```python
from build123d import *

# Parameters (mm, degrees)
BOSS_EXTRUDE1_DEPTH     = 47.498
CUT_EXTRUDE3_DEPTH      = 115.467517244
CUT_EXTRUDE3_DEPTH_BACK = 115.467517244
SKETCH2_R               = 2.413
SKETCH2_4_R             = 2.413
CUT_EXTRUDE4_DEPTH      = 115.467517244
SKETCH6_R               = 12.7
BOSS_EXTRUDE5_DEPTH     = 25.4
SKETCH6_6_R             = 12.7
BOSS_EXTRUDE6_DEPTH     = 25.4
SKETCH8_R               = 2.413
CUT_EXTRUDE5_DEPTH      = 25.4
SKETCH9_R               = 2.413
CUT_EXTRUDE6_DEPTH      = 25.4


with BuildPart() as part:
    # Sketch1 → Boss-Extrude1 (new body)
    with BuildSketch(Plane(origin=(0, 0, 0), x_dir=(1, 0, 0), z_dir=(0, 1, 0))):
        with BuildLine():
            Line((0, 0), (0, 63.5))
            Line((0, 63.5), (12.7, 63.5))
            ThreePointArc((12.7, 63.5), (41.275, 34.925), (69.85, 63.5))
            Line((69.85, 63.5), (82.55, 63.5))
            Line((82.55, 63.5), (82.55, 0))
            Line((82.55, 0), (0, 0))
        make_face()
    extrude(amount=BOSS_EXTRUDE1_DEPTH)

    # Sketch2 → Cut-Extrude3 (cut, two sides: drawn at the far end of the back side and taken through both)
    with BuildSketch(Plane(origin=(0, 47.498, 0), x_dir=(1, 0, 0), z_dir=(0, 1, 0)).offset(-CUT_EXTRUDE3_DEPTH_BACK)):
        with Locations(Location((15.875, 12.7, 0), (0, 0, 90))):
            Circle(SKETCH2_R)
    extrude(amount=CUT_EXTRUDE3_DEPTH + CUT_EXTRUDE3_DEPTH_BACK, mode=Mode.SUBTRACT)

    # Sketch2_4 → Cut-Extrude4 (cut, through all)
    with BuildSketch(Plane(origin=(0, 47.498, 0), x_dir=(1, 0, 0), z_dir=(0, 1, 0))):
        with Locations(Location((15.875, 12.7, 0), (0, 0, 90))):
            Circle(SKETCH2_4_R)
        with Locations(Location((41.275, 12.7, 0), (0, 0, 270))):
            Circle(SKETCH2_4_R)
        with Locations(Location((66.675, 12.7, 0), (0, 0, 270))):
            Circle(SKETCH2_4_R)
    extrude(amount=-CUT_EXTRUDE4_DEPTH, mode=Mode.SUBTRACT)

    # Sketch6 → Boss-Extrude5 (add)
    with BuildSketch(Plane(origin=(0, 0, -63.5), x_dir=(-1, 0, 0), z_dir=(0, 0, -1))):
        with Locations((-82.55, 23.749)):
            Circle(SKETCH6_R)
    extrude(amount=-BOSS_EXTRUDE5_DEPTH)

    # Sketch6_6 → Boss-Extrude6 (add)
    with BuildSketch(Plane(origin=(0, 0, -63.5), x_dir=(-1, 0, 0), z_dir=(0, 0, -1))):
        with Locations((0, 24.290625464)):
            Circle(SKETCH6_6_R)
        with Locations((-82.55, 23.749)):
            Circle(SKETCH6_6_R)
    extrude(amount=-BOSS_EXTRUDE6_DEPTH)

    # Sketch8 → Cut-Extrude5 (cut)
    with BuildSketch(Plane(origin=(0, 0, -63.5), x_dir=(-1, 0, 0), z_dir=(0, 0, -1))):
        with Locations((-88.9, 23.749)):
            Circle(SKETCH8_R)
    extrude(amount=-CUT_EXTRUDE5_DEPTH, mode=Mode.SUBTRACT)

    # Sketch9 → Cut-Extrude6 (cut)
    with BuildSketch(Plane(origin=(0, 0, -63.5), x_dir=(-1, 0, 0), z_dir=(0, 0, -1))):
        with Locations((6.296749676, 24.139451287)):
            Circle(SKETCH9_R)
    extrude(amount=-CUT_EXTRUDE6_DEPTH, mode=Mode.SUBTRACT)


solid = part.part
```
Source: CAD feature listing. Evaluate the final solid. Frame: model axes, mm. A direction names the side the tool comes from. Round coordinates to 2 decimals unless told otherwise and drop trailing zeros. Loops run counter-clockwise (first coordinate to the right, second up) from the corner with the lowest first, then second, coordinate; pieces in that order, holes last. Notation, with made-up numbers: M 13.5,-26 L 41.5,-26 A31 ccw 41.5,12 Z; hole C 1.5,77.25 d4. An arc over 180 degrees is marked long. Use a Markdown table: item, result. Add a question column.
1. Line query: line 1 (X direction, y = 30, z = -12.7); line 2 (X direction, y = 2.5, z = -5.5); line 3 (Z direction, x = 17, y = 32). Output: solid intervals per line, ascending.
2. Contact query for flat-ended pins moving along their axis: P1, Ø10, axis at x = 13.5, y = 24.5, coming from the -Z side; P2, Ø14, axis at y = 15, z = -44, coming from the -X side; P3, Ø1.5, axis at y = 37, z = -22, coming from the -X side; P4, Ø10, axis at y = 24, z = -9, coming from the +X side. Output: stop coordinate, or through.
3. Reachability of faces 4 (the flat face through (82.55, 23, -25)), 5 (the flat face through (0, 23, -24)), 6 (the flat face through (-3, 24, -38.1)), 7 (the flat face through (86, 24, -38.1)) from +Z, -Z, +X, -X, +Y, -Y: full face, straight path, thin tool, end or side. Return the list, or none.
4. Mould query, pull axis X, two halves, no side actions, for faces 1 (the flat face through (42, 0, -25)), 2 (the cylindrical face through (95.247, 24.028, -50.978)), 3 (the cylindrical face through (-4.52, 25.77, -50.98)). Classes: pulls with the +X half, pulls with the -X half, needs draft (parallel to the pull), parting line crosses it, or undercut.
5. Section query D-D on y = 45. Return the cut outline in (x, z) (3 decimals), then the cut area to 3 significant figures.
6. Section query A-A on z = -12.7. Return the cut outline in (x, y).
7. Section query C-C on x = 88.9. Return the cut outline in (y, z), then the cut area to 3 significant figures.
8. Section query B-B on z = -45.5. Return the cut outline in (x, y).
Reported:
| question | item | result |
|---|---|---|
| 1 | line 1 | x = 0 to 13.46, 18.29 to 38.86, 43.69 to 64.26, 69.09 to 82.55 |
| 1 | line 2 | x = 0 to 82.55 |
| 1 | line 3 | z = -48.43 to -14.83, -10.57 to 0 |
| 2 | P1 | stops at z = -63.5 |
| 2 | P2 | stops at x = -12.49 |
| 2 | P3 | stops at x = 0 |
| 2 | P4 | stops at x = 82.55 |
| 3 | face 4 | +Z, +X |
| 3 | face 5 | +Z, -X |
| 3 | face 6 | +Z, -X, +Y, -Y |
| 3 | face 7 | +Z, +X, +Y, -Y |
| 4 | face 1 | needs draft |
| 4 | face 2 | pulls with the +X half |
| 4 | face 3 | undercut |
| 5 | outline | M 0,-63.5 L 12.7,-63.5 A28.575 cw 69.85,-63.5 L 82.55,-63.5 L 82.55,0 L 0,0 Z; hole C 15.875,-12.7 d4.826; hole C 41.275,-12.7 d4.826; hole C 66.675,-12.7 d4.826 |
| 5 | area | 3,900 mm² |
| 6 | outline | M 0,0 L 13.46,0 L 13.46,47.5 L 0,47.5 Z; M 18.29,0 L 38.86,0 L 38.86,47.5 L 18.29,47.5 Z; M 43.69,0 L 64.26,0 L 64.26,47.5 L 43.69,47.5 Z; M 69.09,0 L 82.55,0 L 82.55,47.5 L 69.09,47.5 Z |
| 7 | outline | M 12.75,-63.5 L 21.34,-63.5 L 21.34,-38.1 L 12.75,-38.1 Z; M 26.16,-63.5 L 34.75,-63.5 L 34.75,-38.1 L 26.16,-38.1 Z |
| 7 | area | 436 mm² |
| 8 | outline | M 0,0 L 19.08,0 L 19.08,47.5 L 0,47.5 L 0,36.99 A12.7 ccw 0,11.59 Z; M 63.47,0 L 82.55,0 L 82.55,11.05 A12.7 ccw 82.55,36.45 L 82.55,47.5 L 63.47,47.5 Z; hole C -6.3,24.14 d4.83; hole C 88.9,23.75 d4.83 |
